Geometry check sheet. Reference: the model listing, model coordinates, mm. A direction names the side the tool comes from. Round coordinates to 2 decimals unless told otherwise and drop trailing zeros. Write each loop counter-clockwise with the first axis right and the second up, starting at its lowest first coordinate (ties: lowest second). Pieces come first, ordered by that corner, then holes.
Item 1: Scan lines: probe 1 along X at (y, z) = (0.5, 12); probe 2 along Z at (x, y) = (-24, -10.75). Record each from-to range of solid material in increasing order.
Item 2: Draft check along Z on faces 4 (the face through (10.5, 0, 39)), 5 (the face through (0, 0, 0)), 6 (the face through (7, 11, 5)). Enter one of: pulls with the +Z half, pulls with the -Z half, needs draft (parallel to the pull), parting line crosses it, or undercut.
Item 3: Depth check by flat-ended pin: P1, Ø5, axis at y = 10, z = 17, coming from the -X side; P2, Ø13, axis at y = 5.5, z = 24.5, coming from the +X side; P3, Ø10, axis at x = -20, y = -5.5, coming from the -Z side. Enter the tip coordinate at first touch or a pass-through.
Item 4: Cross-section at B-B (z = 12.5). Enter the section's corners in (x, y), then the cut area to 3 significant figures.
Item 5: Cross-section at A-A (x = 16.5). Enter the section's corners in (y, z), then the cut area to 3 significant figures.
Item 6: Access from +Z, -Z, +X, -X, +Y, -Y to the whole of each face (thin tool, end or side, straight path). Record for faces 1 (the face through (0, -10.5, 39)), 2 (the face through (-7, 11, 5)), 3 (the face through (13, 0, 22)).
Item 7: Cross-section at D-D (y = -2.75). Enter the section's corners in (x, z).
Item 8: Cross-section at C-C (z = 4.5). Enter the section's corners in (x, y).
from build123d import *

# Parameters (mm, degrees)
F0_W      = 26
F0_H      = 26
F0_W_2    = 16
F0_H_2    = 16
F1_DEPTH  = 2
F2_DEPTH  = 40
F3_W      = 26
F3_H      = 26
F3_W_2    = 18
F3_H_2    = 18
F4_DEPTH  = 4
F7_W      = 14
F7_H      = 6
F8_DEPTH  = 15.3
F9_W      = 15
F9_H      = 26
F10_DEPTH = 2
F11_W     = 15
F11_H     = 26
F12_DEPTH = 2
F13_W     = 21
F13_H     = 21
F14_DEPTH = 10


with BuildPart() as f1:
    # F0 (on Top) → F1 (new body)
    with BuildSketch(Plane.XY):
        Rectangle(F0_W, F0_H)
        Rectangle(F0_W_2, F0_H_2, mode=Mode.SUBTRACT)
        Rectangle(F0_W_2, F0_H_2)
    extrude(amount=F1_DEPTH)

    # F0 (on Top) → F2 (join)
    with BuildSketch(Plane.XY):
        Rectangle(F0_W, F0_H)
        Rectangle(F0_W_2, F0_H_2, mode=Mode.SUBTRACT)
    extrude(amount=F2_DEPTH)

    # F3 (on face) → F4 (join)
    with BuildSketch(Plane.XY.offset(40)):
        Rectangle(F3_W, F3_H)
        Rectangle(F3_W_2, F3_H_2, mode=Mode.SUBTRACT)
    extrude(amount=F4_DEPTH)

    # F7 (on face) → F8 (cut)
    with BuildSketch(Plane(origin=(0, 13, 0), x_dir=(-1, 0, 0), z_dir=(0, 1, 0))):
        with Locations((0, 5)):
            Rectangle(F7_W, F7_H)
    extrude(amount=-F8_DEPTH, mode=Mode.SUBTRACT)

    # F9 (on face) → F10 (join)
    with BuildSketch(Plane.XY.offset(44)):
        with Locations((-20.5, 0)):
            Rectangle(F9_W, F9_H)
        with Locations((20.5, 0)):
            Rectangle(F9_W, F9_H)
    extrude(amount=-F10_DEPTH)

    # F11 (on face) → F12 (join)
    with BuildSketch(Plane.XY):
        with Locations((-20.5, 0)):
            Rectangle(F11_W, F11_H)
        with Locations((20.5, 0)):
            Rectangle(F11_W, F11_H)
    extrude(amount=F12_DEPTH)

    # F13 (on face) → F14 (cut)
    with BuildSketch(Plane.XY.offset(44)):
        Rectangle(F13_W, F13_H)
    extrude(amount=-F14_DEPTH, mode=Mode.SUBTRACT)


solid = f1.part
Resolved:
1. probe 1: x = -13 to -8, 8 to 13
1. probe 2: z = 0 to 2, 42 to 44
2. face 4: needs draft
2. face 5: pulls with the -Z half
2. face 6: undercut
3. P1: stops at x = -13
3. P2: stops at x = 13
3. P3: stops at z = 0
4. outline: (-13, -13) - (13, -13) - (13, 13) - (-13, 13) - close; hole (-8, -8) - (8, -8) - (8, 8) - (-8, 8) - close
4. area: 420 mm2
5. outline: (-13, 0) - (13, 0) - (13, 2) - (-13, 2) - close; (-13, 42) - (13, 42) - (13, 44) - (-13, 44) - close
5. area: 104 mm2
6. face 1: +Z
6. face 2: +Y
6. face 3: +X, +Y, -Y
7. outline: (-28, 0) - (28, 0) - (28, 2) - (13, 2) - (13, 42) - (28, 42) - (28, 44) - (10.5, 44) - (10.5, 34) - (8, 34) - (8, 2) - (-8, 2) - (-8, 34) - (-10.5, 34) - (-10.5, 44) - (-28, 44) - (-28, 42) - (-13, 42) - (-13, 2) - (-28, 2) - close
8. outline: (-13, -13) - (13, -13) - (13, 13) - (7, 13) - (7, 8) - (8, 8) - (8, -8) - (-8, -8) - (-8, 8) - (-7, 8) - (-7, 13) - (-13, 13) - close
